```python
from build123d import *

# Parameters (mm, degrees)
CUT_EXTRUDE1_DEPTH      = 10
CUT_EXTRUDE1_DEPTH_BACK = 10
SKETCH2_R               = 2
SKETCH2_R_2             = 2.107972828


with BuildPart() as part:
    # Sketch1 → Revolve1 (revolve)
    with BuildSketch(Plane.XY, mode=Mode.PRIVATE) as revolve1_sk:
        Polygon((0, 0), (50, 0), (57.761374705, 0), (57.761374705, 5), (49.761374705, 5), (49.761374705, 10), (0, 10), (0, 5), (-8, 5), (-8, 0), align=None)
    revolve(revolve1_sk.sketch.rotate(Axis((0, 0, 0), (1, 0, 0)), 90), axis=Axis((0, 0, 0), (1, 0, 0)))

    # Sketch2 → Cut-Extrude1 (cut, two sides: drawn at the far end of the back side and taken through both)
    with BuildSketch(Plane(origin=(0, 0, 0), x_dir=(1, 0, 0), z_dir=(0, 1, 0)).offset(-CUT_EXTRUDE1_DEPTH_BACK)):
        with Locations(Location((-4, 0, 0), (0, 0, 270))):
            Circle(SKETCH2_R)
        with Locations(Location((53.652209211, 0, 0), (0, 0, 270))):
            Circle(SKETCH2_R_2)
    extrude(amount=CUT_EXTRUDE1_DEPTH + CUT_EXTRUDE1_DEPTH_BACK, mode=Mode.SUBTRACT)


solid = part.part
```
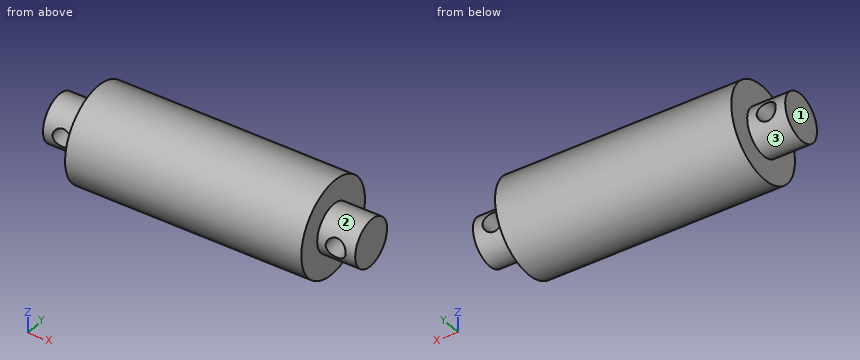
CAD build for the part. Positions are in the model's coordinates, mm. Face numbers are marked on the shaded views. A direction names the side the tool comes from. Give positions to 0.01 mm unless a question says otherwise; leave off trailing zeros. Loops run counter-clockwise (first coordinate to the right, second up) from the corner with the lowest first, then second, coordinate; pieces in that order, holes last. Notation, with made-up numbers: (30.5, 82) -> (40.5, 82) arc R22 ccw to (40.5, 113) -> close; hole circle Ø5 at (36, 80). An arc over 180 degrees is marked (long way). Use a Markdown table: item, result.
1. Slice it at B-B (y = 1). List the corners of the cut face in (x, z).
Check result:
| item | result |
|---|---|
| outline | (-8, -4.9) -> (0, -4.9) -> (0, -9.95) -> (49.76, -9.95) -> (49.76, -4.9) -> (57.76, -4.9) -> (57.76, 4.9) -> (49.76, 4.9) -> (49.76, 9.95) -> (0, 9.95) -> (0, 4.9) -> (-8, 4.9) -> close; hole circle Ø4 at (-4, 0); hole circle Ø4.22 at (53.65, 0) |
2. Which spindle directions (+Z, -Z, +X, -X, +Y, -Y) get a long thin tool onto all of the face, cutting with end or side? Do the marked faces 1, 2 and 3. Say none if no direction does.
Check result:
| item | result |
|---|---|
| face 1 | +Z, -Z, -X, +Y, -Y |
| face 2 | +X |
| face 3 | -X |
3. Wall check: L1, parallel to X at y = -2, z = 0; L2, parallel to Y at x = 18.5, z = 0.25; L3, parallel to Z at x = 54, y = 0.25. Give the ranges that are in metal, low to high. Write a range as [from, to].
Check result:
| item | result |
|---|---|
| L1 | x = [-8, -6], [-2, 51.54], [55.76, 57.76] |
| L2 | y = [-10, 10] |
| L3 | z = [-4.99, -2.08], [2.08, 4.99] |
4. Flat gauge pins, fed straight in: pin 1 (4 mm diameter, centred on y = 6, z = 8, fed in from -X); pin 2 (10 mm diameter, centred on x = 15, z = 3.5, fed in from -Y); pin 3 (4.5 mm diameter, centred on x = -4, z = 0, fed in from +Y); pin 4 (1 mm diameter, centred on x = 8.5, y = 7, fed in from +Z). Where does each tip first touch, or does it go through?
Check result:
| item | result |
|---|---|
| pin 1 | stops at x = 0 |
| pin 2 | stops at y = -10 |
| pin 3 | stops at y = 5 |
| pin 4 | stops at z = 7.6 |
5. Slice it at D-D (z = 8). List the corners of the cut face in (x, y), plus the area to 3 significant figures.
Check result:
| item | result |
|---|---|
| outline | (0, -6) -> (49.76, -6) -> (49.76, 6) -> (0, 6) -> close |
| area | 597 mm^2 |
6. Slice it at C-C (x = -4). List the corners of the cut face in (y, z), plus the area to 3 significant figures.
Check result:
| item | result |
|---|---|
| outline | (-4.58, -2) arc R5 ccw to (4.58, -2) -> close; (-4.58, 2) -> (4.58, 2) arc R5 ccw to start |
| area | 39.6 mm^2 |
7. Slice it at A-A (z = 0). List the corners of the cut face in (x, y), plus the area to 3 significant figures.
Check result:
| item | result |
|---|---|
| outline | (-8, -5) -> (-6, -5) -> (-6, 5) -> (-8, 5) -> close; (-2, -5) -> (0, -5) -> (0, -10) -> (49.76, -10) -> (49.76, -5) -> (51.54, -5) -> (51.54, 5) -> (49.76, 5) -> (49.76, 10) -> (0, 10) -> (0, 5) -> (-2, 5) -> close; (55.76, -5) -> (57.76, -5) -> (57.76, 5) -> (55.76, 5) -> close |
| area | 1,070 mm^2 |
